Read the model definition and answer for the solid it produces. Units are mm, in the model's axes. A direction names the side the tool comes from. Give positions to 0.01 mm unless a question says otherwise; leave off trailing zeros. Order: outer loops, then holes, each group sorted by start corner. A loop starts at its lowest first (then second) coordinate and runs counter-clockwise, first axis right, second up.
Autodesk Inventor part; units mm, degrees
ref_plane "YZ Plane" through (0, 0, 0) normal (1, 0, 0) x (0, 1, 0)
ref_plane "XZ Plane" through (0, 0, 0) normal (0, 1, 0) x (-1, 0, 0)
ref_plane "XY Plane" through (0, 0, 0) normal (0, 0, 1) x (1, 0, 0)
sketch "Sketch1" plane through (0, 0, 0) normal (0, 1, 0) x (-1, 0, 0)
  circle A0 centre (0, 0) radius 50
  circle A1 centre (0, 0) radius 40
  line L0 (-5, -42.5) -> (5, -42.5)
  line L1 (5, -42.5) -> (5, 42.5)
  line L2 (5, 42.5) -> (-5, 42.5)
  line L3 (-5, 42.5) -> (-5, -42.5)
  line L4 (-5, -42.5) -> (5, 42.5) construction
  line L5 (5, -42.5) -> (-5, 42.5) construction
  line L6 (-42.5, -5) -> (42.5, -5)
  line L7 (42.5, -5) -> (42.5, 5)
  line L8 (42.5, 5) -> (-42.5, 5)
  line L9 (-42.5, 5) -> (-42.5, -5)
  line L10 (-42.5, -5) -> (42.5, 5) construction
  line L11 (42.5, -5) -> (-42.5, 5) construction
  point P0 (5, -5)
  point P1 (39.6863, -5)
  point P2 (5, -39.6863)
  point P3 (-5, 5)
  point P4 (-39.6863, 5)
  point P5 (-5, 39.6863)
  point P6 (-5, -5)
  point P7 (-5, -39.6863)
  point P8 (-39.6863, -5)
  point P9 (5, 5)
  point P10 (5, 39.6863)
  point P11 (39.6863, 5)
  dimension "d0" = 100
  dimension "d1" = 80
  dimension "d2" = 10
  dimension "d3" = 85
  dimension "d4" = 85
extrude "Extrusion1" add sketch "Sketch1" along normal blind 8 contours A0 | A1 L6 L1 L8 | A1 L8 L7 L6 | L1 L8 L3 A1 | A1 L3 L2 L1 | L1 L6 L3 L8 | L1 L0 L3 A1 | A1 L3 L6 L1 | L3 L6 A1 L8 | A1 L6 L9 L8
sketch "Sketch2" plane through (0, 8, 0) normal (0, 1, 0) x (1, 0, 0)
  point P0 (0, 0)
  point P1 (-8, 0)
  point P2 (0, 0)
  point P3 (0, -8)
  point P4 (8, 0)
  point P5 (0, 8)
  dimension "d7" = 8
  dimension "d40" = 360
hole "Hole1" at (-8, 8, 0) at (0, 8, -8) at (8, 8, 0) at (0, 8, 8) at (0, 8, 0) direction (0, -1, 0) diameter 5.1 end through all counterbore diameter 6.8 counterbore depth 1
sketch "Sketch6" plane through (0, 0, 0) normal (0, -1, 0) x (1, 0, 0)
  circle A0 centre (0, 8) radius 3.4
  circle A1 centre (8, 0) radius 3.4
  circle A2 centre (0, 0) radius 3.4
  circle A3 centre (-8, 0) radius 3.4
  circle A4 centre (0, -8) radius 3.4
extrude "Extrusion4" cut sketch "Sketch6" against normal blind 1
sketch "Sketch8" plane through (0, 0, 0) normal (0, -1, 0) x (1, 0, 0)
  circle A0 centre (0, 0) radius 50
  circle A1 centre (0, 0) radius 49
  dimension "d45" = 1
extrude "Extrusion5" add sketch "Sketch8" against normal blind 110
sketch "Sketch5" plane through (0, 0, 0) normal (0, -1, 0) x (1, 0, 0)
  circle A0 centre (0, 0) radius 14.6259
  circle A1 centre (0, 0) radius 68.9057
properties part number "Test_base"
1) Given pin 1 (1.5 mm diameter, centred on x = -4, y = 46.5, fed in from -Z); pin 2 (9 mm diameter, centred on x = -8, z = 0, fed in from +Y); pin 3 (1 mm diameter, centred on y = 51.5, z = 18, fed in from +X), each flat-ended and moving along its own axis, determine where each tip first touches the part or whether it passes through.
Final values:
pin 1: stops at z = -49.89
pin 2: stops at y = 8
pin 3: stops at x = 46.84
2) The part is cut by section C-C on x = 0. Count the separate pieces of the cut face and the enclosed holes in it, and give its area (3 significant figures).
Final values:
separate pieces: 4
enclosed holes: 0
area: 871 mm2
3) The part is cut by section B-B on y = 23.5. Determine the outline of the cut face in (x, z).
Final values:
outline: circle Ø100 at (0, 0); hole circle Ø98 at (0, 0)
4) A tool of negligible diameter and unlimited length cuts with its end or side. For faces 1 (the face through (-22, 4, -5)), 2 (the face through (0, 1, -5)), 3 (the face through (11.32, 7.49, -0.74)), from which of +Z, -Z, +X, -X, +Y, -Y can it reach the whole face along a straight path? Write none if from no direction.
Final values:
face 1: +Y, -Y
face 2: -Y
face 3: +Y
5) The part is cut by section D-D on z = -32.5. Determine the outline of the cut face in (x, y).
Final values:
outline: (-38, 0) - (-23.32, 0) - (-23.32, 8) - (-36.67, 8) - (-36.67, 110) - (-38, 110) - close; (-5, 0) - (5, 0) - (5, 8) - (-5, 8) - close; (23.32, 0) - (38, 0) - (38, 110) - (36.67, 110) - (36.67, 8) - (23.32, 8) - close
6) For a pull along Z with two mould halves and no side action, classify faces 4 (the face through (0.977, 3.958, -5.644)), 5 (the face through (1, 0, 12)) as released by +Z, released by -Z, zero draft, split by the parting line, or undercut.
Final values:
face 4: undercut
face 5: zero draft
7) The part is cut by section A-A on z = -8. Determine the outline of the cut face in (x, y), and give its area (3 significant figures).
Final values:
outline: (-49.36, 0) - (-39.19, 0) - (-39.19, 8) - (-48.34, 8) - (-48.34, 110) - (-49.36, 110) - close; (-5, 0) - (-3.4, 0) - (-3.4, 1) - (-2.55, 1) - (-2.55, 7) - (-3.4, 7) - (-3.4, 8) - (-5, 8) - close; (2.55, 1) - (3.4, 1) - (3.4, 0) - (5, 0) - (5, 8) - (3.4, 8) - (3.4, 7) - (2.55, 7) - close; (39.19, 0) - (49.36, 0) - (49.36, 110) - (48.34, 110) - (48.34, 8) - (39.19, 8) - close
area: 405 mm2
8) Consider L1, parallel to Z at x = 0, y = 0.75; L2, parallel to X at y = 3, z = 0; L3, parallel to X at y = 3.9, z = 8. Determine where each line is inside the solid, lowest interval first.
Final values:
L1: z = -50 to -11.4, -4.6 to -3.4, 3.4 to 4.6, 11.4 to 50
L2: x = -50 to -10.55, -5.45 to -2.55, 2.55 to 5.45, 10.55 to 50
L3: x = -49.36 to -39.19, -5 to -2.55, 2.55 to 5, 39.19 to 49.36
